from build123d import *

# Parameters (mm, degrees)
F0_W     = 20
F0_H     = 40
F1_DEPTH = 70
F2_R     = 2.5
F3_DEPTH = 20.001
F4_W     = 10
F4_H     = 30
F5_DEPTH = 70.001


with BuildPart() as f1:
    # F0 (on Front) → F1 (new body)
    with BuildSketch(Plane.XZ):
        with Locations((10, 20)):
            Rectangle(F0_W, F0_H)
    extrude(amount=F1_DEPTH)

    # F2 (on face) → F3 (cut, through all)
    with BuildSketch(Plane.YZ.offset(20)):
        with Locations((-35, 25)):
            Circle(F2_R)
    extrude(amount=-F3_DEPTH, mode=Mode.SUBTRACT)

    # F4 (on face) → F5 (cut, through all)
    with BuildSketch(Plane.XZ.offset(70)):
        with Locations((10, 20)):
            Rectangle(F4_W, F4_H)
    extrude(amount=-F5_DEPTH, mode=Mode.SUBTRACT)


solid = f1.part
Verification items for the finished model (mm, model axes). A direction names the side the tool comes from. Give positions to 0.01 mm unless a question says otherwise; leave off trailing zeros. Order: outer loops, then holes, each group sorted by start corner. A loop starts at its lowest first (then second) coordinate and runs counter-clockwise, first axis right, second up. Notation, with made-up numbers: M -13.75,-22.5 L 30.25,-22.5 A8 cw 30.25,-12.5 Z; hole C 59.25,13 d1. An arc over 180 degrees is marked long. Answer as a JSON object with one key per item and string values. Group by question number.
1) Access from +Z, -Z, +X, -X, +Y, -Y to the whole of each face (thin tool, end or side, straight path). Record for faces 1 (the face through (10, -35, 5)), 2 (the face through (3, -70, 20)).
2) Cross-section at C-C (x = 11.25). Enter the section's corners in (y, z), then the cut area to 3 significant figures.
3) Mould release check, pull along X, two halves, no side actions. Record for faces 3 (the face through (0, -35, 20)), 4 (the face through (2.54, -33.66, 27.11)), 5 (the face through (10, -35, 35)): released by +X, released by -X, zero draft, split by the parting line, or undercut.
4) Scan lines: line 1 along X through (y, z) = (-41, 25.5); line 2 along Z through (x, y) = (14.75, -43); line 3 along Z through (x, y) = (2.95, -35). Record each from-to range of solid material in increasing order. Write a range as [from, to].
5) Depth check by flat-ended pin: pin 1 Ø5 at (x, y) = (13, -55.5) entering from -Z. Enter the tip coordinate at first touch or a pass-through.
6) Cross-section at B-B (z = 31). Enter the section's corners in (x, y), then the cut area to 3 significant figures.
7) Cross-section at D-D (z = 25). Enter the section's corners in (x, y).
8) Cross-section at A-A (y = -35). Enter the section's corners in (x, z).
Result sheet:
{
 "1": {"face 1": "+Y, -Y", "face 2": "+Z, -Z, +X, -X, -Y"},
 "2": {"outline": "M -70,0 L 0,0 L 0,5 L -70,5 Z; M -70,35 L 0,35 L 0,40 L -70,40 Z", "area": "700 mm2"},
 "3": {"face 3": "released by -X", "face 4": "zero draft", "face 5": "undercut"},
 "4": {"line 1": "x = [0, 5], [15, 20]", "line 2": "z = [0, 5], [35, 40]", "line 3": "z = [0, 22.5], [27.5, 40]"},
 "5": {"pin 1": "stops at z = 0"},
 "6": {"outline": "M 0,-70 L 5,-70 L 5,0 L 0,0 Z; M 15,-70 L 20,-70 L 20,0 L 15,0 Z", "area": "700 mm2"},
 "7": {"outline": "M 0,-70 L 5,-70 L 5,-37.5 L 0,-37.5 Z; M 0,-32.5 L 5,-32.5 L 5,0 L 0,0 Z; M 15,-70 L 20,-70 L 20,-37.5 L 15,-37.5 Z; M 15,-32.5 L 20,-32.5 L 20,0 L 15,0 Z"},
 "8": {"outline": "M 0,0 L 20,0 L 20,22.5 L 15,22.5 L 15,5 L 5,5 L 5,22.5 L 0,22.5 Z; M 0,27.5 L 5,27.5 L 5,35 L 15,35 L 15,27.5 L 20,27.5 L 20,40 L 0,40 Z"}
}
